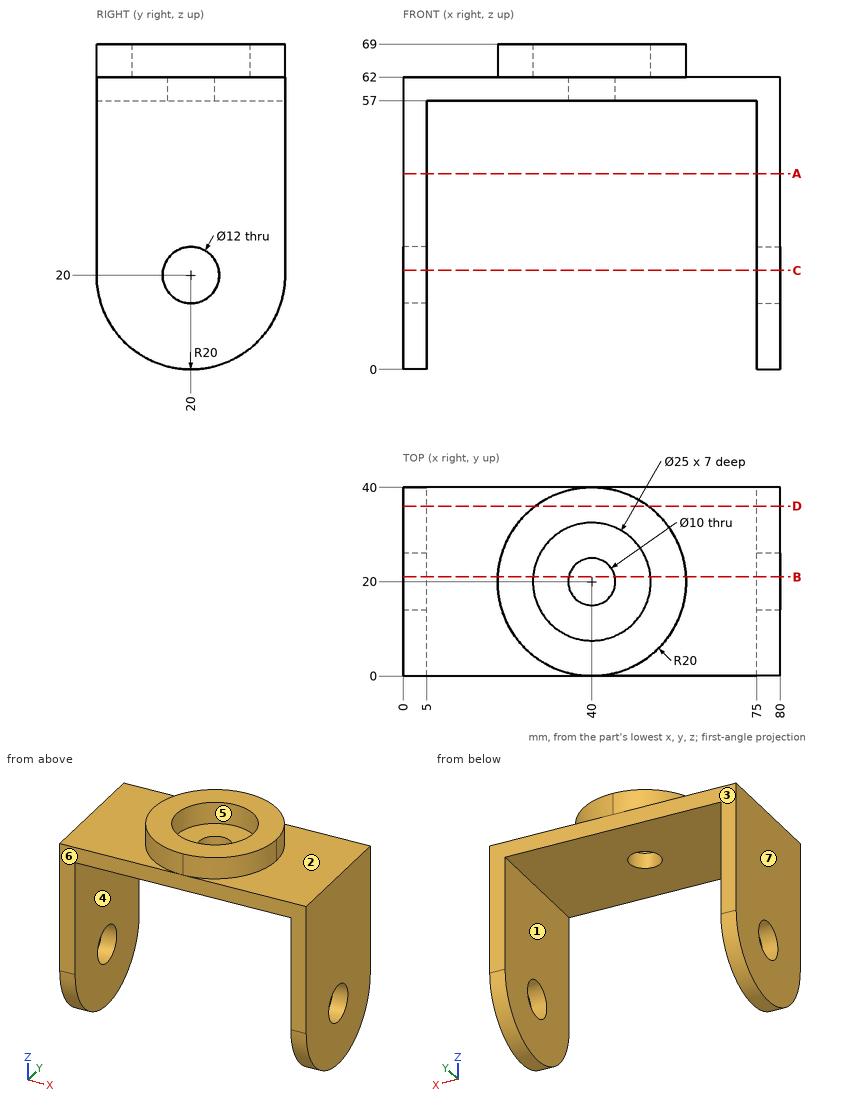
Design review of the part shown in the three views and the two pictorial views. Dimensions are in mm from the part's minimum x, y and z. A direction names the side the tool comes from. Coordinates: 2 decimals unless noted, no trailing zeros. Order: outer loops, then holes, each group sorted by start corner. A loop starts at its lowest first (then second) coordinate and runs counter-clockwise, first axis right, second up.
1) Take a section at A-A, the plane z = 41.5. Give the boundary of the cut face in (x, y).
2) Take a section at D-D, the plane y = 36. Give the boundary of the cut face in (x, z), and give its area (3 significant figures).
3) Clearance check with flat-ended pins moving along their axes: pin 1 (11 mm diameter, centred on y = 20, z = 20, fed in from +X); pin 2 (6 mm diameter, centred on x = 10.5, y = 19.5, fed in from +Z); pin 3 (20 mm diameter, centred on x = 38.5, y = 25.5, fed in from +Z); pin 4 (12 mm diameter, centred on x = 44, y = 23, fed in from -Z). State where each tip first meets the part, or that it passes through.
4) Mouldability with a two-part tool opening along X and no side actions: class the marked faces 4, 5, 6 and 7 as +X half, -X half, draft (parallel to the pull), parting line (faces both ways), or undercut.
5) Take a section at B-B, the plane y = 21. Give the boundary of the cut face in (x, z), and give its area (3 significant figures).
6) Take a section at C-C, the plane z = 21. Give the boundary of the cut face in (x, y).
7) For the marked faces 1, 2 and 3, list the 3-axis set-ups (+Z, -Z, +X, -X, +Y, -Y) from which the entire face can be reached by the end or side of a thin tool; tool diameter is ignored.
8) Wall thickness on line 1 along X through (y, z) = (21, 40.5); line 2 along Y through (x, z) = (40, 66); line 3 along Y through (x, z) = (40, 60.35): over which ranges is each line inside the solid? List them lowest first.
Returned:
1. outline: (0, 0) - (5, 0) - (5, 40) - (0, 40) - close; (75, 0) - (80, 0) - (80, 40) - (75, 40) - close
2. outline: (0, 8) - (5, 8) - (5, 57) - (75, 57) - (75, 8) - (80, 8) - (80, 62) - (52, 62) - (52, 69) - (28, 69) - (28, 62) - (0, 62) - close
2. area: 1,060 mm2
3. pin 1: passes through
3. pin 2: stops at z = 62
3. pin 3: stops at z = 69
3. pin 4: stops at z = 57
4. face 4: undercut
4. face 5: undercut
4. face 6: draft
4. face 7: -X half
5. outline: (0, 0.03) - (5, 0.03) - (5, 14.08) - (0, 14.08) - close; (0, 25.92) - (5, 25.92) - (5, 57) - (35.1, 57) - (35.1, 62) - (27.54, 62) - (27.54, 69) - (20.03, 69) - (20.03, 62) - (0, 62) - close; (44.9, 57) - (75, 57) - (75, 25.92) - (80, 25.92) - (80, 62) - (59.97, 62) - (59.97, 69) - (52.46, 69) - (52.46, 62) - (44.9, 62) - close; (75, 0.03) - (80, 0.03) - (80, 14.08) - (75, 14.08) - close
5. area: 908 mm2
6. outline: (0, 0) - (5, 0) - (5, 14.08) - (0, 14.08) - close; (0, 25.92) - (5, 25.92) - (5, 40) - (0, 40) - close; (75, 0) - (80, 0) - (80, 14.08) - (75, 14.08) - close; (75, 25.92) - (80, 25.92) - (80, 40) - (75, 40) - close
7. face 1: -Z, +Y, -Y
7. face 2: +Z, +X
7. face 3: +Z, -Z, +X, -X, +Y
8. line 1: x = 0 to 5, 75 to 80
8. line 2: y = 0 to 7.5, 32.5 to 40
8. line 3: y = 0 to 15, 25 to 40
